CAD build for the part. Positions are in the model's coordinates, mm. Face numbers are marked on the shaded views. Coordinates: 2 decimals unless noted, no trailing zeros. Order: outer loops, then holes, each group sorted by start corner. A loop starts at its lowest first (then second) coordinate and runs counter-clockwise, first axis right, second up. Notation, with made-up numbers: M -30.75,80.5 L 21.25,80.5 A16 ccw 21.25,94.5 Z; hole C 89,-20.75 d5. An arc over 180 degrees is marked long. One line per item, written item: value.
from build123d import *

# Parameters (mm, degrees)
F0_W     = 76.2
F0_H     = 19.05
F1_DEPTH = 19.05
F3_D     = 12.7
F5_D     = 12.7
F6_R     = 7.62


with BuildPart() as f1:
    # F0 (on Top) → F1 (new body)
    with BuildSketch(Plane.XY):
        with Locations((9.621889, -4.491718)):
            Rectangle(F0_W, F0_H)
    extrude(amount=F1_DEPTH)

    # F3 (through all)
    with Locations(Plane(origin=(0, 5.033282, 0), x_dir=(-1, 0, 0), z_dir=(0, 1, 0))):
        with Locations((18.953111, 9.525)):
            Hole(F3_D / 2)

    # F5 (through all)
    with Locations(Plane.XZ.offset(14.016718)):
        with Locations((38.196889, 9.525)):
            Hole(F5_D / 2)

    # F6
    f6_edges = [f1.edges().sort_by_distance(p)[0] for p in [
        (47.721889, -4.491718, 19.05),
        (47.721889, -4.491718, 0),
        (-28.478111, -4.491718, 19.05),
        (-28.478111, -4.491718, 0),
    ]]
    fillet(f6_edges, radius=F6_R)


solid = f1.part
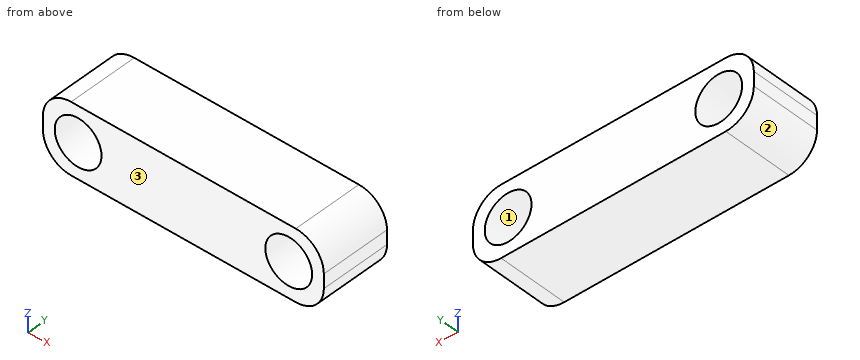
Q1. Drill centre lines: line 1 along X through (y, z) = (-1, 9.75); line 2 along X through (y, z) = (0.5, 6.25); line 3 along Z through (x, y) = (35.5, 1.5). Where is each one in solid material? Low to high.
Recorded:
line 1: x = -28.48 to -25.3, -12.61 to 31.85, 44.54 to 47.72
line 2: x = -28.35 to -24.39, -13.51 to 32.76, 43.64 to 47.6
line 3: z = 0 to 3.78, 15.27 to 19.05
Q2. Slice it at B-B (z = 6.25). List the corners of the cut face in (x, y), plus the area to 3 significant figures.
Recorded:
outline: M -28.35,-14.02 L -24.39,-14.02 L -24.39,5.03 L -28.35,5.03 Z; M -13.51,-14.02 L 32.76,-14.02 L 32.76,5.03 L -13.51,5.03 Z; M 43.64,-14.02 L 47.6,-14.02 L 47.6,5.03 L 43.64,5.03 Z
area: 1,030 mm^2
Q3. Pin check, flat tips, straight feed: pin 1 Ø1 at (x, z) = (-19, 15.5) entering from -Y; pin 2 Ø6 at (y, z) = (-4, 16) entering from -X; pin 3 Ø3 at (y, z) = (1.5, 15) entering from -X. Stop position of each tip, or through.
Recorded:
pin 1: stops at y = -14.02
pin 2: stops at x = -28.31
pin 3: stops at x = -28.19
Q4. Slice it at C-C (y = -6.75). List the corners of the cut face in (x, z) (3 decimals).
Recorded:
outline: M -28.478,7.62 A7.62 ccw -20.858,0 L 40.102,0 A7.62 ccw 47.722,7.62 L 47.722,11.43 A7.62 ccw 40.102,19.05 L -20.858,19.05 A7.62 ccw -28.478,11.43 Z; hole C -18.953,9.525 d12.7; hole C 38.197,9.525 d12.7
Q5. Mould opens along X. For the marked faces 1, 2 and 3 say: released by +X, released by -X, zero draft, split by the parting line, or undercut.
Recorded:
face 1: undercut
face 2: released by -X
face 3: zero draft
Q6. Slice it at D-D (z = 10.25). List the corners of the cut face in (x, y).
Recorded:
outline: M -28.48,-14.02 L -25.26,-14.02 L -25.26,5.03 L -28.48,5.03 Z; M -12.64,-14.02 L 31.89,-14.02 L 31.89,5.03 L -12.64,5.03 Z; M 44.51,-14.02 L 47.72,-14.02 L 47.72,5.03 L 44.51,5.03 Z
Q7. Slice it at A-A (x = 36). List the corners of the cut face in (y, z).
Recorded:
outline: M -14.02,0 L 5.03,0 L 5.03,3.57 L -14.02,3.57 Z; M -14.02,15.48 L 5.03,15.48 L 5.03,19.05 L -14.02,19.05 Z
